Verification items for the finished model (mm, model axes). Face numbers are marked on the shaded views. A direction names the side the tool comes from. Coordinates: 2 decimals unless noted, no trailing zeros. Loops run counter-clockwise (first coordinate to the right, second up) from the corner with the lowest first, then second, coordinate; pieces in that order, holes last.
Q1. Material ranges on probe 1 along Z at (x, y) = (0.75, 3); probe 2 along Z at (x, y) = (-0.5, -0.5); probe 3 along Y at (x, z) = (-0.25, 11.75), recorded low to high.
Q2. Sectioned sample at B-B (z = 12.75). Enter the section's corners in (x, y).
Q3. Sectioned sample at A-A (z = 22). Enter the section's corners in (x, y).
Q4. Go/stop test with flat-tipped pins: P1, Ø1, axis at x = 0, y = -0.5, coming from the +Z side; P2, Ø2, axis at x = -1.5, z = 13.5, coming from the +Y side; P3, Ø1.5, axis at x = 2, z = 17, coming from the -Y side. Record where each tip stops, or that it passes through.
Q5. Access from +Z, -Z, +X, -X, +Y, -Y to the whole of each face (thin tool, end or side, straight path). Record for the marked faces 1 and 2.
```python
from build123d import *

# Parameters (mm, degrees)
F0_R     = 4.25
F1_DEPTH = 19
F2_R     = 1
F3_R     = 1.5
F4_DEPTH = 1
F5_R     = 0.5
F7_R     = 0.5
F8_DEPTH = 8
F9_R     = 0.25


with BuildPart() as f1:
    # F0 (on Top) → F1 (new body)
    with BuildSketch(Plane.XY):
        Circle(F0_R)
    extrude(amount=F1_DEPTH)

    # F2
    f2_edges = [f1.edges().sort_by_distance(p)[0] for p in [
        (-4.25, 0, 19),
        (-4.25, 0, 0),
    ]]
    fillet(f2_edges, radius=F2_R)

    # F3 (on face) → F4 (join)
    with BuildSketch(Plane.XY.offset(19)):
        Circle(F3_R)
    extrude(amount=F4_DEPTH)

    # F5
    f5_edges = [f1.edges().sort_by_distance(p)[0] for p in [
        (-1.5, 0, 20),
    ]]
    fillet(f5_edges, radius=F5_R)

    # F7 (on face) → F8 (join)
    with BuildSketch(Plane.XY.offset(20)):
        Circle(F7_R)
    extrude(amount=F8_DEPTH)

    # F9
    f9_edges = [f1.edges().sort_by_distance(p)[0] for p in [
        (-0.5, 0, 28),
    ]]
    fillet(f9_edges, radius=F9_R)


solid = f1.part
```
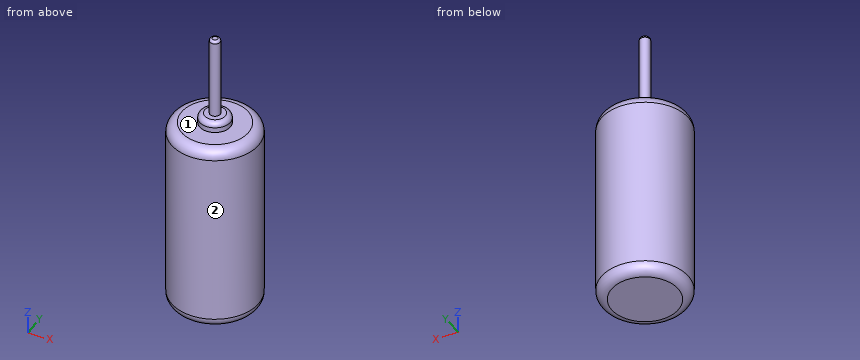
Geometry check:
1. probe 1: z = 0 to 19
1. probe 2: z = 0 to 20
1. probe 3: y = -4.24 to 4.24
2. outline: circle Ø8.5 at (0, 0)
3. outline: circle Ø1 at (0, 0)
4. P1: stops at z = 28
4. P2: stops at y = 4.22
4. P3: stops at y = -4.06
5. face 1: +Z
5. face 2: +Z, -Z
